Part model, mm, in its own coordinate system. A direction names the side the tool comes from. Coordinates: 2 decimals unless noted, no trailing zeros. Loops run counter-clockwise (first coordinate to the right, second up) from the corner with the lowest first, then second, coordinate; pieces in that order, holes last. Notation, with made-up numbers: M 19.5,-31 L 56.5,-31 A29 cw 56.5,-10 Z; hole C 39,-21.5 d10. An arc over 180 degrees is marked long. Use a Markdown table: item, result. Add a question column.
1) Pull direction Y, two halves, no side cores. Call faces 4 (the cylindrical face through (-101.347, 33.594, 16.78)), 5 (the cylindrical face through (-92.042, 32.181, 16.78)), 6 (the flat face through (-99, 28, 91.186)): released by +Y, released by -Y, zero draft, split by the parting line, or undercut.
2) Band-saw the part on B-B (y = 39.5). List the corners of the cut face in (x, z).
3) Pin check, flat tips, straight feed: pin 1 Ø4 at (x, z) = (-85.5, 32.5) entering from -Y; pin 2 Ø19.5 at (x, y) = (-80.69, 27.49) entering from +Z; pin 3 Ø3 at (x, z) = (24.5, 36.5) entering from +Y. Stop position of each tip, or through.
4) Band-saw the part on D-D (z = 32). List the corners of the cut face in (x, y), plus the area to 3 significant figures.
5) Band-saw the part on A-A (x = -45.5). List the corners of the cut face in (y, z).
6) Wall check: probe 1 along Z at (x, y) = (-19.5, 41.5); probe 2 along X at (y, z) = (29.5, 100.5); probe 3 along X at (y, z) = (27, 114.5). Give the ranges that are in metal, low to high. Write a range as from..to.
7) Band-saw the part on C-C (x = -73). List the corners of the cut face in (y, z).
8) Tool access for faces 1 (the flat face through (-29.667, 5.322, 16.78)), 2 (the flat face through (-33, 52.39, 107)), 3 (the cylindrical face through (-65.86, 21.34, 106.9)): list every direction of +Z, -Z, +X, -X, +Y, -Y with a clear straight run to the whole face (end or side of a thin tool).
from build123d import *

# Parameters (mm, degrees)
F0_R      = 25.332369153
F1_DEPTH  = 122.428
F3_DEPTH  = 34.036
F4_R      = 25.1663808995
F5_DEPTH  = 34.036
F6_W      = 99.9408867977
F6_H      = 49.807743342
F7_DEPTH  = 31.496
F9_DEPTH  = 31.242
F11_R     = 15.866808683
F12_DEPTH = 52.832
F10_R     = 16.051664823
F13_DEPTH = 70.104
F14_R     = 17.5666522391
F15_DEPTH = 262.382


with BuildPart() as f1:
    # F0 (on Top) → F1 (new body)
    with BuildSketch(Plane.XY):
        with Locations((21.7129960656, 27.794552967)):
            Circle(F0_R)
    extrude(amount=F1_DEPTH)

    # F2 (on face) → F3 (join)
    with BuildSketch(Plane(origin=(0, 0, 0), x_dir=(1, 0, 0), z_dir=(0, 0, -1))):
        with BuildLine():
            ThreePointArc((24.2469048948, -42.8027561924), (33.3369903631, -37.6205193104), (36.9336024271, -27.794552967))
            ThreePointArc((36.9336024271, -27.794552967), (33.3369903631, -17.9685866235), (24.2469048948, -12.7863497415))
            Line((24.2469048948, -12.7863497415), (24.2469048948, -42.8027561924))
        make_face()
        with BuildLine():
            Line((24.2469048948, -42.8027561924), (24.2469048948, -12.7863497415))
            ThreePointArc((24.2469048948, -12.7863497415), (6.4923897041, -27.794552967), (24.2469048948, -42.8027561924))
        make_face()
        with BuildLine():
            ThreePointArc((24.2469048948, -42.8027561924), (6.4923897041, -27.794552967), (24.2469048948, -12.7863497415))
            Line((24.2469048948, -12.7863497415), (24.2469048948, -2.5892314465))
            Line((24.2469048948, -2.5892314465), (-77.2918909788, -7.7366237529))
            Line((-77.2918909788, -7.7366237529), (-75.0896409154, -58.021184057))
            Line((-75.0896409154, -58.021184057), (24.2469048948, -52.9998744874))
            Line((24.2469048948, -52.9998744874), (24.2469048948, -42.8027561924))
        make_face()
        with BuildLine():
            ThreePointArc((21.7336893247, -53.1269136681), (-3.4898764651, -30.3527052507), (16.6431184636, -2.9746966417))
            Line((16.6431184636, -2.9746966417), (-77.2918909788, -7.7366237529))
            Line((-77.2918909788, -7.7366237529), (-75.0896409154, -58.021184057))
            Line((-75.0896409154, -58.021184057), (21.7336893247, -53.1269136681))
        make_face()
    extrude(amount=-F3_DEPTH)

    # F4 (on face) → F5 (join)
    with BuildSketch(Plane(origin=(0, 0, 0), x_dir=(1, 0, 0), z_dir=(0, 0, -1))):
        with Locations((-76.1907659471, -32.8789039049)):
            Circle(F4_R)
    extrude(amount=-F5_DEPTH)

    # F6 (on face) → F7 (join)
    with BuildSketch(Plane.XY.offset(122.428)):
        with Locations((-30.7190240909, 27.4859363282)):
            Rectangle(F6_W, F6_H)
    extrude(amount=-F7_DEPTH)

    # F8 (on face) → F9 (join)
    with BuildSketch(Plane.XY.offset(122.428)):
        with BuildLine():
            Line((-80.6894674897, 2.5820646572), (-80.6894674897, 52.3898079991))
            ThreePointArc((-80.6894674897, 52.3898079991), (-105.5933391607, 27.4859363282), (-80.6894674897, 2.5820646572))
        make_face()
    extrude(amount=-F9_DEPTH)

    # F11 (on face) → F12 (cut)
    with BuildSketch(Plane(origin=(0, 0, 0), x_dir=(1, 0, 0), z_dir=(0, 0, -1))):
        with Locations((-76.1907659471, -32.8789039049)):
            Circle(F11_R)
    extrude(amount=-F12_DEPTH, mode=Mode.SUBTRACT)

    # F10 (on face) → F13 (cut)
    with BuildSketch(Plane.XY.offset(122.428)):
        with Locations((-80.6894674897, 27.4859363282)):
            Circle(F10_R)
    extrude(amount=-F13_DEPTH, mode=Mode.SUBTRACT)

    # F14 (on face) → F15 (cut)
    with BuildSketch(Plane.XY.offset(122.428)):
        with Locations((21.7129960656, 27.794552967)):
            Circle(F14_R)
    extrude(amount=-F15_DEPTH, mode=Mode.SUBTRACT)


solid = f1.part
Entries:
| question | item | result |
|---|---|---|
| 1 | face 4 | split by the parting line |
| 1 | face 5 | undercut |
| 1 | face 6 | zero draft |
| 2 | outline | M -102.5,91.19 L -91.33,91.19 L -91.33,122.43 L -102.5,122.43 Z; M -100.47,0 L -90.61,0 L -90.61,34.04 L -100.47,34.04 Z; M -70.04,90.93 L -0.75,90.93 L -0.75,34.04 L -61.77,34.04 L -61.77,0 L 8.61,0 L 8.61,122.43 L -70.04,122.43 Z; M 34.81,0 L 44.18,0 L 44.18,122.43 L 34.81,122.43 Z |
| 3 | pin 1 | y = 8.8 |
| 3 | pin 2 | z = 34.04 |
| 3 | pin 3 | y = 53.09 |
| 4 | outline | M -77.29,7.74 L 16.64,2.97 A25.33 ccw long 21.73,53.13 L -74.75,58 A25.17 ccw long Z; hole C -76.19,32.88 d31.73; hole C 21.71,27.79 d35.13 |
| 4 | area | 5,180 mm2 |
| 5 | outline | M 2.58,90.93 L 52.39,90.93 L 52.39,122.43 L 2.58,122.43 Z; M 6.12,0 L 56.53,0 L 56.53,34.04 L 6.12,34.04 Z |
| 6 | probe 1 | 0..34.04, 90.93..122.43 |
| 6 | probe 2 | -105.51..-96.61, -64.76..4.23, 39.2..46.99 |
| 6 | probe 3 | -105.59..-96.73, -64.65..4.16, 39.26..47.03 |
| 7 | outline | M 2.58,90.93 L 13.4,90.93 L 13.4,122.43 L 2.58,122.43 Z; M 7.52,0 L 17.34,0 L 17.34,34.04 L 7.52,34.04 Z; M 41.58,90.93 L 52.39,90.93 L 52.39,122.43 L 41.58,122.43 Z; M 48.42,0 L 57.92,0 L 57.92,34.04 L 48.42,34.04 Z |
| 8 | face 1 | -Z, -X, -Y |
| 8 | face 2 | +Z, -X, +Y |
| 8 | face 3 | +Z |
